Read the model definition and answer for the solid it produces. Units are mm, in the model's axes. Face numbers are marked on the shaded views. A direction names the side the tool comes from. Coordinates: 2 decimals unless noted, no trailing zeros. Write each loop counter-clockwise with the first axis right and the second up, starting at its lowest first coordinate (ties: lowest second). Pieces come first, ordered by that corner, then holes. Notation, with made-up numbers: (34.25, 5) -> (80.25, 5) arc R16 cw to (80.25, 24) -> close; hole circle Ø1 at (52, -39). An arc over 180 degrees is marked (long way). One line per item, written item: value. Start each with the question number.
1. For the marked faces 4 and 5, determine the directions among +Z, -Z, +X, -X, +Y, -Y from which every point of the face is accessible in a straight line to the end or side of a thin tool.
2. For a pull along Y with two mould halves and no side action, classify the marked faces 1, 2 and 3 as pulls with the +Y half, pulls with the -Y half, needs draft (parallel to the pull), parting line crosses it, or undercut.
3. Find section A-A, the plane z = 2.75. Write down the section's boundary in (x, y).
4. Given P1, Ø3, axis at y = -22.5, z = 4, coming from the -X side; P2, Ø3, axis at x = -11.69, y = 6.75, coming from the +Z side; P3, Ø1.5, axis at y = 2.5, z = 3.5, coming from the +X side; P4, Ø1, axis at y = -30.5, z = 3.5, coming from the +X side, each flat-ended and moving along its own axis, determine where each tip first touches the part or whether it passes through.
5. Find section C-C, the plane x = 0. Write down the section's boundary in (y, z).
6. Find section B-B, the plane y = -9. Write down the section's boundary in (x, z).
7. Find section D-D, the plane y = 6.75. Write down the section's boundary in (x, z), and give its area (3 significant figures).
8. Consider line 1 along Y through (x, z) = (0, 3.65); line 2 along Y through (x, z) = (2, 0.95); line 3 along Y through (x, z) = (1, 1.7). Determine where each line is inside the solid, lowest interval first.
```python
from build123d import *

# Parameters (mm, degrees)
EXTRUDE_1_DEPTH     = 5
SKETCH_3_R          = 2.5
CUT_EXTRUDE_1_DEPTH = 24
SKETCH_4_R          = 1.525
CUT_EXTRUDE_2_DEPTH = 5
SKETCH_5_R          = 2.5
CUT_EXTRUDE_3_DEPTH = 5
FILLET_1_R          = 5
SKETCH_6_R          = 1.3
SKETCH_6_R_2        = 10
CUT_EXTRUDE_4_DEPTH = 10
SKETCH_7_R          = 16
SKETCH_7_R_2        = 10
SKETCH_7_R_3        = 1.3
EXTRUDE_2_DEPTH     = 5
FILLET_2_R          = 5


with BuildPart() as part:
    # 草图1 → 凸台-拉伸1 (new body)
    with BuildSketch(Plane.XY):
        with BuildLine():
            Line((5, -8.077747211), (5, -45))
            ThreePointArc((5, -45), (0, -50), (-5, -45))
            Line((-5, -45), (-5, -8.077747211))
            ThreePointArc((-5, -8.077747211), (0, 9.5), (5, -8.077747211))
        make_face()
    extrude(amount=EXTRUDE_1_DEPTH)

    # 草图3 → 切除-拉伸1 (cut)
    with BuildSketch(Plane.XY.offset(5)):
        with Locations((0, -45)):
            Circle(SKETCH_3_R)
    extrude(amount=-CUT_EXTRUDE_1_DEPTH, mode=Mode.SUBTRACT)

    # 草图4 → 切除-拉伸2 (cut)
    with BuildSketch(Plane.XY.offset(5)):
        with Locations((0, 6.25)):
            Circle(SKETCH_4_R)
        with Locations((0, -6.25)):
            Circle(SKETCH_4_R)
    extrude(amount=-CUT_EXTRUDE_2_DEPTH, mode=Mode.SUBTRACT)

    # 草图5 → 切除-拉伸3 (cut)
    with BuildSketch(Plane.XY.offset(5)):
        Circle(SKETCH_5_R)
    extrude(amount=-CUT_EXTRUDE_3_DEPTH, mode=Mode.SUBTRACT)

    # 圆角1
    fillet_1_edges = [part.edges().sort_by_distance(p)[0] for p in [
        (-5, -8.077747211, 2.5),
        (5, -8.077747211, 2.5),
    ]]
    fillet(fillet_1_edges, radius=FILLET_1_R)

    # 草图6 → 切除-拉伸4 (cut)
    with BuildSketch(Plane.XY.offset(5)):
        with Locations((0, -13.5)):
            Circle(SKETCH_6_R)
        Circle(SKETCH_6_R_2)
    extrude(amount=-CUT_EXTRUDE_4_DEPTH, mode=Mode.SUBTRACT)

    # 草图7 → 凸台-拉伸2 (add)
    with BuildSketch(Plane.XY.offset(5)):
        Circle(SKETCH_7_R)
        Circle(SKETCH_7_R_2, mode=Mode.SUBTRACT)
        with Locations((11.691342951, 6.75)):
            Circle(SKETCH_7_R_3, mode=Mode.SUBTRACT)
        with Locations((-11.691342951, 6.75)):
            Circle(SKETCH_7_R_3, mode=Mode.SUBTRACT)
        with Locations((0, -13.5)):
            Circle(SKETCH_7_R_3, mode=Mode.SUBTRACT)
    extrude(amount=-EXTRUDE_2_DEPTH)

    # 圆角2
    fillet_2_edges = [part.edges().sort_by_distance(p)[0] for p in [
        (5, -15.198684154, 2.5),
        (-5, -15.198684154, 2.5),
    ]]
    fillet(fillet_2_edges, radius=FILLET_2_R)


solid = part.part
```
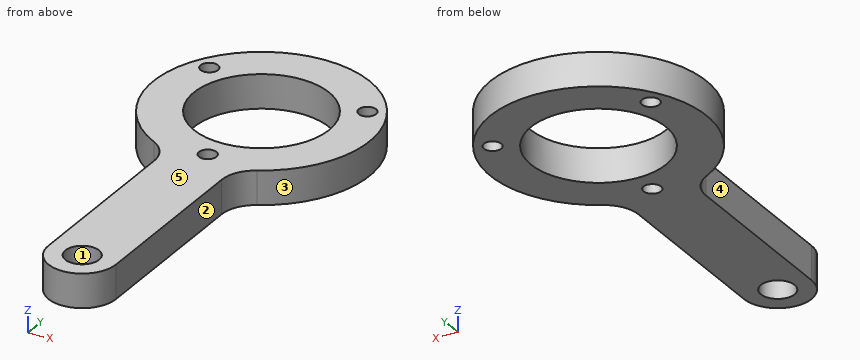
Answer block:
1. face 4: +Z, -Z, -X, -Y
1. face 5: +Z, +X, -X, +Y, -Y
2. face 1: undercut
2. face 2: needs draft
2. face 3: parting line crosses it
3. outline: (-7.62, -14.07) arc R5 cw to (-5, -18.47) -> (-5, -45) arc R5 ccw to (5, -45) -> (5, -18.47) arc R5 cw to (7.62, -14.07) arc R16 ccw (long way) to start; hole circle Ø2.6 at (-11.69, 6.75); hole circle Ø20 at (0, 0); hole circle Ø5 at (0, -45); hole circle Ø2.6 at (0, -13.5); hole circle Ø2.6 at (11.69, 6.75)
4. P1: stops at x = -5
4. P2: stops at z = 5
4. P3: stops at x = 15.9
4. P4: stops at x = 5
5. outline: (-50, 0) -> (-47.5, 0) -> (-47.5, 5) -> (-50, 5) -> close; (-42.5, 0) -> (-14.8, 0) -> (-14.8, 5) -> (-42.5, 5) -> close; (-12.2, 0) -> (-10, 0) -> (-10, 5) -> (-12.2, 5) -> close; (10, 0) -> (16, 0) -> (16, 5) -> (10, 5) -> close
6. outline: (-13.23, 0) -> (-4.36, 0) -> (-4.36, 5) -> (-13.23, 5) -> close; (4.36, 0) -> (13.23, 0) -> (13.23, 5) -> (4.36, 5) -> close
7. outline: (-14.51, 0) -> (-12.99, 0) -> (-12.99, 5) -> (-14.51, 5) -> close; (-10.39, 0) -> (-7.38, 0) -> (-7.38, 5) -> (-10.39, 5) -> close; (7.38, 0) -> (10.39, 0) -> (10.39, 5) -> (7.38, 5) -> close; (12.99, 0) -> (14.51, 0) -> (14.51, 5) -> (12.99, 5) -> close
7. area: 45.3 mm2
8. line 1: y = -50 to -47.5, -42.5 to -14.8, -12.2 to -10, 10 to 16
8. line 2: y = -49.58 to -46.5, -43.5 to -9.8, 9.8 to 15.87
8. line 3: y = -49.9 to -47.29, -42.71 to -14.33, -12.67 to -9.95, 9.95 to 15.97
